Check sheet for the modelled part. Datum: model origin and axes. Units: mm. A direction names the side the tool comes from. Coordinates: 2 decimals unless noted, no trailing zeros. Write each loop counter-clockwise with the first axis right and the second up, starting at its lowest first coordinate (ties: lowest second). Pieces come first, ordered by that corner, then holes. Notation, with made-up numbers: (68, 27) -> (101, 27) arc R20 ccw to (101, 47) -> close; hole circle Ø7 at (74, 7.5). An arc over 180 degrees is marked (long way). One line per item, written item: value. Start each with the question number.
1) Draft check along X on faces 1 (the flat face through (-25.256, -31.551, 35.916)), 2 (the conical face through (14.18, 4.47, 7.5)), 3 (the flat face through (25.256, 31.551, 35.916)), 4 (the cylindrical face through (0, -63, 36)). Enter one of: +X half, -X half, draft (parallel to the pull), parting line (faces both ways), or undercut.
2) Sectioned sample at B-B on y = 0. Enter the section's corners in (x, z).
3) Scan lines: line 1 along Y through (x, z) = (0, 35); line 2 along Y through (x, z) = (2, 35); line 3 along Z through (x, y) = (-18, 30.5). Record each from-to range of solid material in increasing order. Write a range as [from, to].
4) Sectioned sample at A-A on x = 0. Enter the section's corners in (y, z).
5) Sectioned sample at D-D on y = -44. Enter the section's corners in (x, z).
6) Sectioned sample at C-C on z = 19.5. Enter the section's corners in (x, y).
7) Set-up check for faces 5 (the cylindrical face through (-35, 0, 36)), 6 (the cylindrical face through (25.865, 10.724, 14.79)): record each of +Z, -Z, +X, -X, +Y, -Y from which the full face is reachable in a straight line by a thin tool's end or side.
8) Gauge pin test, flat ends, axial feed: P1, Ø6, axis at x = 12.5, y = 34, coming from the -Z side; P2, Ø4, axis at x = 8.5, z = 35, coming from the -Y side; P3, Ø21, axis at x = 0, y = 12, coming from the -Z side. Record the tip position at first contact, or that the pin passes through.
```python
from build123d import *

# Parameters (mm, degrees)
F0_R     = 7
F0_R_2   = 14
F1_DEPTH = 42
F2_R     = 7
F2_R_2   = 28
F3_DEPTH = 30
F4_SIZE2 = 13.856406
F4_SIZE  = 8


with BuildPart() as f1:
    # F0 (on Top) → F1 (new body)
    with BuildSketch(Plane.XY):
        with BuildLine():
            Line((32.603934, 12.727273), (17.699279, 50.909091))
            ThreePointArc((17.699279, 50.909091), (0, 63), (-17.699279, 50.909091))
            Line((-17.699279, 50.909091), (-32.603934, 12.727273))
            ThreePointArc((-32.603934, 12.727273), (-35, 0), (-32.603934, -12.727273))
            Line((-32.603934, -12.727273), (-17.699279, -50.909091))
            ThreePointArc((-17.699279, -50.909091), (0, -63), (17.699279, -50.909091))
            Line((17.699279, -50.909091), (32.603934, -12.727273))
            ThreePointArc((32.603934, -12.727273), (35, 0), (32.603934, 12.727273))
        make_face()
        with Locations((0, -44)):
            Circle(F0_R, mode=Mode.SUBTRACT)
        Circle(F0_R_2, mode=Mode.SUBTRACT)
        with Locations((0, 44)):
            Circle(F0_R, mode=Mode.SUBTRACT)
    extrude(amount=F1_DEPTH)

    # F2 (on face) → F3 (cut)
    with BuildSketch(Plane(origin=(0, 0, 0), x_dir=(1, 0, 0), z_dir=(0, 0, -1))):
        with BuildLine():
            ThreePointArc((-17.699279, -50.909091), (0, -63), (17.699279, -50.909091))
            Line((17.699279, -50.909091), (32.603934, -12.727273))
            ThreePointArc((32.603934, -12.727273), (35, 0), (32.603934, 12.727273))
            Line((32.603934, 12.727273), (17.699279, 50.909091))
            ThreePointArc((17.699279, 50.909091), (0, 63), (-17.699279, 50.909091))
            Line((-17.699279, 50.909091), (-32.603934, 12.727273))
            ThreePointArc((-32.603934, 12.727273), (-35, 0), (-32.603934, -12.727273))
            Line((-32.603934, -12.727273), (-17.699279, -50.909091))
        make_face()
        with Locations((0, -44)):
            Circle(F2_R, mode=Mode.SUBTRACT)
        Circle(F2_R_2, mode=Mode.SUBTRACT)
        with Locations((0, 44)):
            Circle(F2_R, mode=Mode.SUBTRACT)
    extrude(amount=-F3_DEPTH, mode=Mode.SUBTRACT)

    # F4
    f4_edges = [f1.edges().sort_by_distance(p)[0] for p in [
        (-14, 0, 0),
    ]]
    chamfer(f4_edges, length=F4_SIZE, length2=F4_SIZE2)


solid = f1.part
```
Answers:
1. face 1: -X half
1. face 2: undercut
1. face 3: +X half
1. face 4: parting line
2. outline: (-35, 30) -> (-28, 30) -> (-28, 0) -> (-27.86, 0) -> (-14, 8) -> (-14, 42) -> (-35, 42) -> close; (14, 8) -> (27.86, 0) -> (28, 0) -> (28, 30) -> (35, 30) -> (35, 42) -> (14, 42) -> close
3. line 1: y = [-63, -51], [-37, -14], [14, 37], [51, 63]
3. line 2: y = [-62.89, -50.71], [-37.29, -13.86], [13.86, 37.29], [50.71, 62.89]
3. line 3: z = [30, 42]
4. outline: (-63, 30) -> (-51, 30) -> (-51, 42) -> (-63, 42) -> close; (-37, 30) -> (-28, 30) -> (-28, 0) -> (-27.86, 0) -> (-14, 8) -> (-14, 42) -> (-37, 42) -> close; (14, 8) -> (27.86, 0) -> (28, 0) -> (28, 30) -> (37, 30) -> (37, 42) -> (14, 42) -> close; (51, 30) -> (63, 30) -> (63, 42) -> (51, 42) -> close
5. outline: (-20.4, 30) -> (-7, 30) -> (-7, 42) -> (-20.4, 42) -> close; (7, 30) -> (20.4, 30) -> (20.4, 42) -> (7, 42) -> close
6. outline: circle Ø56 at (0, 0); hole circle Ø28 at (0, 0)
7. face 5: +Z, -Z, -X
7. face 6: -Z
8. P1: stops at z = 30
8. P2: stops at y = -61.85
8. P3: stops at z = 3.09
